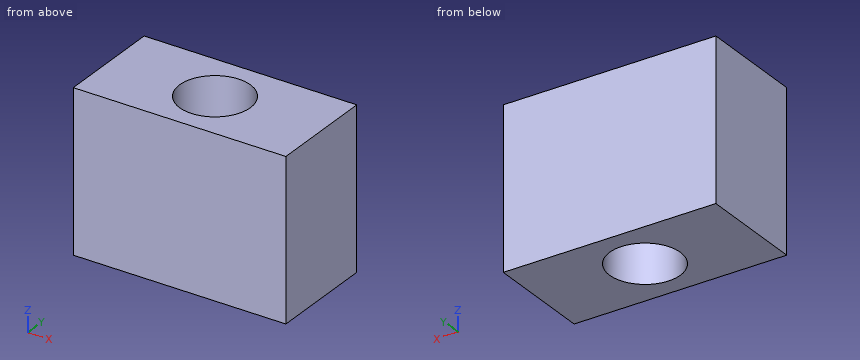
from build123d import *

# Parameters (mm, degrees)
F0_R     = 10
F1_DEPTH = 45


with BuildPart() as f1:
    # F0 (on Top) → F1 (new body)
    with BuildSketch(Plane.XY):
        Polygon((12.5, 30), (-12.5, 30), (-30, 30), (-30, 0), (-12.5, 0), (12.5, 0), (30, 0), (30, 30), align=None)
        with Locations((0, 15)):
            Circle(F0_R, mode=Mode.SUBTRACT)
    extrude(amount=F1_DEPTH)


solid = f1.part
The listing builds one solid part. Answer for the finished solid, in the listing's coordinates (mm). Give positions to 0.01 mm unless a question says otherwise; leave off trailing zeros. Write each loop counter-clockwise with the first axis right and the second up, starting at its lowest first coordinate (ties: lowest second). Pieces come first, ordered by that corner, then holes.
1) Find the intervals of material crossed by L1, parallel to Y at x = 0, z = 21; L2, parallel to X at y = 15.5, z = 16; L3, parallel to X at y = 23.5, z = 6, in increasing order.
2) Section A-A (x = 0) is taken. Write down the section's boundary in (y, z), and give its area (3 significant figures).
3) Section B-B (y = 15) is taken. Write down the section's boundary in (x, z), and give its area (3 significant figures).
4) Section C-C (z = 32.5) is taken. Write down the section's boundary in (x, y).
Response:
1. L1: y = 0 to 5, 25 to 30
1. L2: x = -30 to -9.99, 9.99 to 30
1. L3: x = -30 to -5.27, 5.27 to 30
2. outline: (0, 0) - (5, 0) - (5, 45) - (0, 45) - close; (25, 0) - (30, 0) - (30, 45) - (25, 45) - close
2. area: 450 mm2
3. outline: (-30, 0) - (-10, 0) - (-10, 45) - (-30, 45) - close; (10, 0) - (30, 0) - (30, 45) - (10, 45) - close
3. area: 1,800 mm2
4. outline: (-30, 0) - (30, 0) - (30, 30) - (-30, 30) - close; hole circle Ø20 at (0, 15)
